from build123d import *

# Parameters (mm, degrees)
SALIENTE_EXTRUIR1_DEPTH = 200
CROQUIS5_W              = 40
CROQUIS5_H              = 13
SALIENTE_EXTRUIR4_DEPTH = 13
REDONDEO9_R             = 7
REDONDEO11_R            = 5


with BuildPart() as part:
    # Croquis1 → Saliente-Extruir1 (new body)
    with BuildSketch(Plane(origin=(0, 0, 0), x_dir=(1, 0, 0), z_dir=(0, 1, 0))):
        Polygon((5, 140), (10, 0), (5, 0), (0, 0), (0, 140), align=None)
    extrude(amount=SALIENTE_EXTRUIR1_DEPTH)

    # Croquis5 → Saliente-Extruir4 (add)
    with BuildSketch(Plane.ZY):
        with Locations((-20, 196.5)):
            Rectangle(CROQUIS5_W, CROQUIS5_H)
        with Locations((-20, 3.5)):
            Rectangle(CROQUIS5_W, CROQUIS5_H)
    extrude(amount=-SALIENTE_EXTRUIR4_DEPTH)

    # Redondeo9
    redondeo9_edges = [part.edges().sort_by_distance(p)[0] for p in [
        (13, 203, -20),
        (13, -3, -20),
    ]]
    fillet(redondeo9_edges, radius=REDONDEO9_R)

    # Redondeo11
    redondeo11_edges = [part.edges().sort_by_distance(p)[0] for p in [
        (6.785714286, 0, -90),
        (6.785714286, 200, -90),
    ]]
    fillet(redondeo11_edges, radius=REDONDEO11_R)


solid = part.part
Design review of the part built by this model. Coordinates are the model's own, in mm. A direction names the side the tool comes from. Give positions to 0.01 mm unless a question says otherwise; leave off trailing zeros. Write each loop counter-clockwise with the first axis right and the second up, starting at its lowest first coordinate (ties: lowest second). Pieces come first, ordered by that corner, then holes. Notation, with made-up numbers: M 82.5,85.25 L 137.5,85.25 A22 cw 137.5,114.25 Z; hole C 13,28.25 d3. An arc over 180 degrees is marked long. Return JSON: item names as keys, results as strings. Group by question number.
Item 1: Take a section at A-A (z = -36.5). Give the boundary of the cut face in (x, y), plus the area to 3 significant figures.
Item 2: Take a section at B-B (y = 78.5). Give the boundary of the cut face in (x, z).
Item 3: The part is to be moulded in two halves that separate along Y. For faces 1 (the cylindrical face through (11, 200.9, -19.7)), 2 (the flat face through (5, 99, 0)), 3 (the flat face through (11, 10, -20)), say which applies: pulls with the +Y half, pulls with the -Y half, needs draft (parallel to the pull), parting line crosses it, or undercut.
Item 4: Tool access review of faces 4 (the flat face through (8, 2, -40)), 5 (the flat face through (8, 198, -40)), 6 (the flat face through (11, 190, -20)): name each direction out of +Z, -Z, +X, -X, +Y, -Y from which nothing blocks a thin tool from reaching the whole face with its end or side.
Item 5: Clearance check with flat-ended pins moving along their axes: pin 1 Ø2 at (x, z) = (12, -22.5) entering from -Y; pin 2 Ø3 at (x, z) = (1.5, -83) entering from +Y; pin 3 Ø5 at (x, z) = (3, -110) entering from -Y. State where each tip first meets the part, or that it passes through.
Item 6: Wall thickness on line 1 along Y through (x, z) = (6.5, -15); line 2 along X through (y, z) = (125, -70); line 3 along X through (y, z) = (15.5, -61): over which ranges is each line inside the solid? List them lowest first.
Item 7: Take a section at C-C (z = -12). Give the boundary of the cut face in (x, y).
Return value:
{
 "1": {"outline": "M 0,-3 L 6,-3 A7 ccw 13,4 L 13,10 L 8.7,10 L 8.7,190 L 13,190 L 13,196 A7 ccw 6,203 L 0,203 Z", "area": "1,880 mm2"},
 "2": {"outline": "M 0,-140 L 5,-140 L 10,0 L 0,0 Z"},
 "3": {"face 1": "pulls with the +Y half", "face 2": "needs draft", "face 3": "undercut"},
 "4": {"face 4": "-Z, +X, -Y", "face 5": "-Z, +X, +Y", "face 6": "-Z, +X"},
 "5": {"pin 1": "stops at y = -0.9", "pin 2": "stops at y = 200", "pin 3": "stops at y = 0"},
 "6": {"line 1": "y = -2.98 to 202.98", "line 2": "x = 0 to 7.5", "line 3": "x = 0 to 7.82"},
 "7": {"outline": "M 0,-3 L 6,-3 A7 ccw 13,4 L 13,10 L 9.57,10 L 9.57,190 L 13,190 L 13,196 A7 ccw 6,203 L 0,203 Z"}
}
